Check sheet for the modelled part. Datum: model origin and axes. Units: mm. Face numbers are marked on the shaded views. Round coordinates to 2 decimals unless told otherwise and drop trailing zeros. Loops run counter-clockwise (first coordinate to the right, second up) from the corner with the lowest first, then second, coordinate; pieces in that order, holes last. Notation, with made-up numbers: (67.5, 59) -> (98.5, 59) arc R21 ccw to (98.5, 69) -> close; hole circle Ø1 at (0.5, 23.5). An arc over 180 degrees is marked (long way). One line per item, written item: value. Start each with the question number.
1. Cross-section at B-B on y = -18. Record the cut outline in (x, z).
2. Cross-section at A-A on x = 15. Record the cut outline in (y, z).
3. Go/stop test with a flat-tipped pin: pin 1 (8 mm diameter, centred on x = 56, y = -3.5, fed in from -Z). Record where the tip stops, or that it passes through.
4. Material ranges on L1, parallel to Y at x = 15, z = 3.4; L2, parallel to X at y = -13.5, z = 4.9; L3, parallel to X at y = -7, z = 3.7, recorded low to high.
5. Release check for a two-part mould opening along Y. For the marked faces 1 and 2 record: +Y half, -Y half, draft (parallel to the pull), parting line (faces both ways), or undercut.
6. Cross-section at C-C on z = 3.25. Record the cut outline in (x, y), then the cut area to 3 significant figures.
Autodesk Inventor part; units mm, degrees
ref_plane "YZ Plane" through (0, 0, 0) normal (1, 0, 0) x (0, 1, 0)
ref_plane "XZ Plane" through (0, 0, 0) normal (0, 1, 0) x (-1, 0, 0)
ref_plane "XY Plane" through (0, 0, 0) normal (0, 0, 1) x (1, 0, 0)
sketch "스케치1" plane through (0, 0, 0) normal (0, 0, 1) x (1, 0, 0)
  line L0 (-12.2, 0) -> (71.7, 0)
  line L1 (71.7, 5.8) -> (71.7, 0)
  line L2 (-12.2, 5.8) -> (71.7, 5.8)
  line L3 (-12.2, 5.8) -> (-12.2, 0)
  line L4 (-12.2, 5.8) -> (71.7, 5.8)
  line L5 (71.7, 5.8) -> (71.7, 11.8)
  line L6 (71.7, 11.8) -> (-12.2, 11.8)
  line L7 (-12.2, 11.8) -> (-12.2, 5.8)
  line L8 (-12.2, -46.0408) -> (71.7, -46.0408)
  line L9 (71.7, -40.2408) -> (71.7, -46.0408)
  line L10 (-12.2, -40.2408) -> (71.7, -40.2408)
  line L11 (-12.2, -40.2408) -> (-12.2, -46.0408)
  line L12 (-12.2, -46.0408) -> (71.7, -46.0408)
  line L13 (71.7, -46.0408) -> (71.7, -52.0408)
  line L14 (71.7, -52.0408) -> (-12.2, -52.0408)
  line L15 (-12.2, -52.0408) -> (-12.2, -46.0408)
  line L16 (-12.2, 0) -> (71.7, 0)
  line L17 (71.7, 0) -> (71.7, -40.2408)
  line L18 (71.7, -40.2408) -> (-12.2, -40.2408)
  line L19 (-12.2, -40.2408) -> (-12.2, 0)
  point P0 (0, 0)
  dimension "d0" = 6
  dimension "d3" = 6
extrude "돌출1" add sketch "스케치1" along normal blind 6
sketch "스케치2" plane through (0, 0, 6) normal (0, 0, 1) x (1, 0, 0)
  circle A0 centre (15, -19.9408) radius 14.2
  point P0 (0, 0)
extrude "돌출2" cut sketch "스케치2" against normal blind 6
properties part number "부품72"
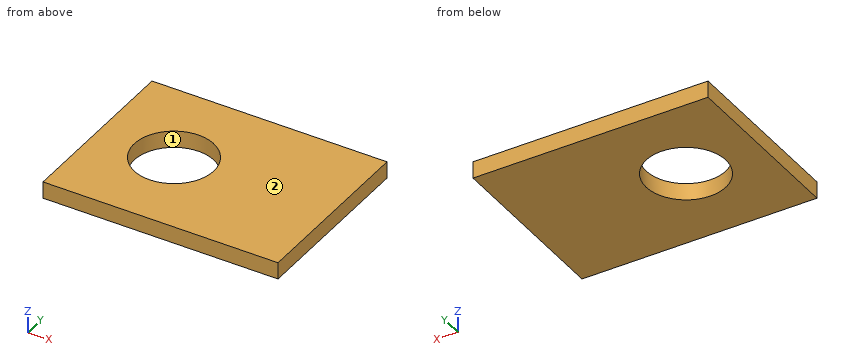
Taken from the geometry:
1. outline: (-12.2, 0) -> (0.93, 0) -> (0.93, 6) -> (-12.2, 6) -> close; (29.07, 0) -> (71.7, 0) -> (71.7, 6) -> (29.07, 6) -> close
2. outline: (-52.04, 0) -> (-34.14, 0) -> (-34.14, 6) -> (-52.04, 6) -> close; (-5.74, 0) -> (11.8, 0) -> (11.8, 6) -> (-5.74, 6) -> close
3. pin 1: stops at z = 0
4. L1: y = -52.04 to -34.14, -5.74 to 11.8
4. L2: x = -12.2 to 2.34, 27.66 to 71.7
4. L3: x = -12.2 to 9.15, 20.85 to 71.7
5. face 1: undercut
5. face 2: draft
6. outline: (-12.2, -52.04) -> (71.7, -52.04) -> (71.7, 11.8) -> (-12.2, 11.8) -> close; hole circle Ø28.4 at (15, -19.94)
6. area: 4,720 mm2
